from build123d import *

# Parameters (mm, degrees)
SKETCH_W      = 150
SKETCH_H      = 10
PAD_DEPTH     = 4
SKETCH001_R   = 5
SKETCH001_R_2 = 4
PAD001_DEPTH  = 8
FILLET_R      = 4.99
SKETCH002_W   = 5.5
SKETCH002_H   = 2.5
POCKET_DEPTH  = 3.5
SKETCH004_W   = 5
SKETCH004_H   = 2
PAD002_DEPTH  = 3
SKETCH005_W   = 5
SKETCH005_H   = 2
PAD003_DEPTH  = 3
SKETCH006_W   = 7
SKETCH006_H   = 10
PAD004_DEPTH  = 1
SKETCH008_R   = 2.5
PAD005_DEPTH  = 15
FILLET001_R   = 2.49


with BuildPart() as part:
    # Sketch → Pad (new body)
    with BuildSketch(Plane.XY):
        Rectangle(SKETCH_W, SKETCH_H)
    extrude(amount=PAD_DEPTH)

    # Sketch001 (on Face6 of Pad) → Pad001 (join)
    with BuildSketch(Plane.XY.offset(4)):
        Circle(SKETCH001_R)
        Circle(SKETCH001_R_2, mode=Mode.SUBTRACT)
        with Locations((60, 0)):
            Circle(SKETCH001_R)
        with Locations((60, 0)):
            Circle(SKETCH001_R_2, mode=Mode.SUBTRACT)
        with Locations((-60, 0)):
            Circle(SKETCH001_R)
        with Locations((-60, 0)):
            Circle(SKETCH001_R_2, mode=Mode.SUBTRACT)
    extrude(amount=PAD001_DEPTH)

    # Fillet
    fillet_edges = [part.edges().sort_by_distance(p)[0] for p in [
        (-75, 5, 2),
        (-75, -5, 2),
        (75, 5, 2),
        (75, -5, 2),
    ]]
    fillet(fillet_edges, radius=FILLET_R)

    # Sketch002 (on Face2 of Fillet) → Pocket (cut)
    with BuildSketch(Plane(origin=(0, 0, 0), x_dir=(1, 0, 0), z_dir=(0, 0, -1))):
        with Locations((-68, 0)):
            Rectangle(SKETCH002_W, SKETCH002_H)
        with Locations((68, 0)):
            Rectangle(SKETCH002_W, SKETCH002_H)
    extrude(amount=-POCKET_DEPTH, mode=Mode.SUBTRACT)

    # Sketch004 (on Face6 of Pocket) → Pad002 (join)
    with BuildSketch(Plane(origin=(0, 5, 0), x_dir=(-1, 0, 0), z_dir=(0, 1, 0))):
        with Locations((-30, 2)):
            Rectangle(SKETCH004_W, SKETCH004_H)
        with Locations((30, 2)):
            Rectangle(SKETCH004_W, SKETCH004_H)
    extrude(amount=PAD002_DEPTH)

    # Sketch005 (on Face7 of Pocket) → Pad003 (join)
    with BuildSketch(Plane.XZ.offset(5)):
        with Locations((-30, 2)):
            Rectangle(SKETCH005_W, SKETCH005_H)
        with Locations((30, 2)):
            Rectangle(SKETCH005_W, SKETCH005_H)
    extrude(amount=PAD003_DEPTH)

    # Sketch006 (on Face22 of Pad003) → Pad004 (join)
    with BuildSketch(Plane.XY.offset(4)):
        with Locations((-30, 0)):
            Rectangle(SKETCH006_W, SKETCH006_H)
        with Locations((30, 0)):
            Rectangle(SKETCH006_W, SKETCH006_H)
    extrude(amount=PAD004_DEPTH)

    # Sketch008 (on Face55 of Pad004) → Pad005 (join)
    with BuildSketch(Plane.XY.offset(5)):
        with Locations((-30, 0)):
            Circle(SKETCH008_R)
        with Locations((30, 0)):
            Circle(SKETCH008_R)
    extrude(amount=PAD005_DEPTH)

    # Fillet001
    fillet001_edges = [part.edges().sort_by_distance(p)[0] for p in [
        (27.5, 0, 20),
        (-32.5, 0, 20),
    ]]
    fillet(fillet001_edges, radius=FILLET001_R)


solid = part.part
Verification items for the finished model (mm, model axes). A direction names the side the tool comes from. Give positions to 0.01 mm unless a question says otherwise; leave off trailing zeros. Loops run counter-clockwise (first coordinate to the right, second up) from the corner with the lowest first, then second, coordinate; pieces in that order, holes last.
1) Thickness scan on line 1 along X through (y, z) = (-0.25, 3.25); line 2 along Y through (x, z) = (-60, 6.25); line 3 along Z through (x, y) = (-35.5, -4.5). Record the ranges inside material, lowest first.
2) Draft check along Y on faces 6 (the flat face through (60, 0, 4)), 7 (the cylindrical face through (-65, 0, 8)), 8 (the flat face through (-1, 0, 0)). Enter one of: pulls with the +Y half, pulls with the -Y half, needs draft (parallel to the pull), parting line crosses it, or undercut.
3) Set-up check for faces 1 (the flat face through (30, -6, 3)), 2 (the flat face through (30, 6, 3)), 3 (the flat face through (-68, 1.25, 2)), 4 (the flat face through (30, 6, 1)), 5 (the cylindrical face through (55, 0, 8)): record each of +Z, -Z, +X, -X, +Y, -Y from which the full face is reachable in a straight line by a thin tool's end or side.
4) Depth check by flat-ended pin: pin 1 Ø5 at (x, y) = (-2, 1) entering from +Z; pin 2 Ø1.6 at (y, z) = (-7, 2.5) entering from +X; pin 3 Ø4 at (y, z) = (2.5, 16) entering from +X. Enter the tip coordinate at first touch or a pass-through.
5) Sectioned sample at A-A, the plane z = 9. Enter the section's corners in (x, y), then the cut area to 3 significant figures.
6) Sectioned sample at B-B, the plane x = 61.5. Enter the section's corners in (y, z).
Answers:
1. line 1: x = -74.99 to -70.75, -65.25 to 65.25, 70.75 to 74.99
1. line 2: y = -5 to -4, 4 to 5
1. line 3: z = 0 to 4
2. face 6: undercut
2. face 7: parting line crosses it
2. face 8: needs draft
3. face 1: +Z, +X, -X, -Y
3. face 2: +Z, +X, -X, +Y
3. face 3: -Z
3. face 4: -Z, +X, -X, +Y
3. face 5: +Z
4. pin 1: stops at z = 12
4. pin 2: stops at x = 32.5
4. pin 3: stops at x = 32.45
5. outline: circle Ø10 at (-60, 0); circle Ø5 at (-30, 0); circle Ø10 at (0, 0); circle Ø5 at (30, 0); circle Ø10 at (60, 0); hole circle Ø8 at (-60, 0); hole circle Ø8 at (0, 0); hole circle Ø8 at (60, 0)
5. area: 124 mm2
6. outline: (-5, 0) - (5, 0) - (5, 4) - (4.77, 4) - (4.77, 12) - (3.71, 12) - (3.71, 4) - (-3.71, 4) - (-3.71, 12) - (-4.77, 12) - (-4.77, 4) - (-5, 4) - close
